```python
from build123d import *

# Parameters (mm, degrees)
CROQUIS1_W              = 237
CROQUIS1_H              = 450
SALIENTE_EXTRUIR1_DEPTH = 10
CROQUIS2_W              = 5
CROQUIS2_H              = 450
SALIENTE_EXTRUIR2_DEPTH = 70
CROQUIS3_R              = 2
CORTAR_EXTRUIR1_DEPTH   = 70
CROQUIS4_W              = 450
CROQUIS4_H              = 70
CORTAR_EXTRUIR2_DEPTH   = 10
CROQUIS5_R              = 10
CORTAR_EXTRUIR4_DEPTH   = 10


with BuildPart() as part:
    # Croquis1 → Saliente-Extruir1 (new body)
    with BuildSketch(Plane(origin=(0, 0, 0), x_dir=(1, 0, 0), z_dir=(0, 1, 0))):
        Rectangle(CROQUIS1_W, CROQUIS1_H)
    extrude(amount=SALIENTE_EXTRUIR1_DEPTH)

    # Croquis2 → Saliente-Extruir2 (add)
    with BuildSketch(Plane.XZ):
        with Locations((-116, 0)):
            Rectangle(CROQUIS2_W, CROQUIS2_H)
    extrude(amount=SALIENTE_EXTRUIR2_DEPTH)

    # Croquis3 → Cortar-Extruir1 (cut)
    with BuildSketch(Plane(origin=(-113.5, 0, 0), x_dir=(0, 0, -1), z_dir=(1, 0, 0))):
        with Locations((-215, -10)):
            Circle(CROQUIS3_R)
        with Locations((215, -10)):
            Circle(CROQUIS3_R)
        with Locations((215, -60)):
            Circle(CROQUIS3_R)
        with Locations((-215, -60)):
            Circle(CROQUIS3_R)
    extrude(amount=-CORTAR_EXTRUIR1_DEPTH, mode=Mode.SUBTRACT)

    # Croquis4 → Cortar-Extruir2 (cut)
    with BuildSketch(Plane(origin=(-113.5, 0, 0), x_dir=(0, 0, -1), z_dir=(1, 0, 0))):
        with Locations((0, -35)):
            Rectangle(CROQUIS4_W, CROQUIS4_H)
    extrude(amount=-CORTAR_EXTRUIR2_DEPTH, mode=Mode.SUBTRACT)

    # Croquis5 → Cortar-Extruir4 (cut)
    with BuildSketch(Plane.XZ):
        with Locations((-98.5, 35.8)):
            Circle(CROQUIS5_R)
    extrude(amount=-CORTAR_EXTRUIR4_DEPTH, mode=Mode.SUBTRACT)


solid = part.part
```
Build history of the part. All positions in model axes, mm. Coordinates: 2 decimals unless noted, no trailing zeros. Write each loop counter-clockwise with the first axis right and the second up, starting at its lowest first coordinate (ties: lowest second). Pieces come first, ordered by that corner, then holes.
1. Band-saw the part on B-B, the plane x = -98.5. Give the cut face in (y, z), and give its area (3 significant figures).
Answer block:
outline: (0, -225) - (10, -225) - (10, 25.8) - (0, 25.8) - close; (0, 45.8) - (10, 45.8) - (10, 225) - (0, 225) - close
area: 4,300 mm2
2. Pull direction Z, two halves, no side cores. Call faces 1 (the flat face through (-2, 5, -225)), 2 (the cylindrical face through (-105.87, 4.93, 42.56)), 3 (the flat face through (-2, 10, -3)): released by +Z, released by -Z, zero draft, split by the parting line, or undercut.
Answer block:
face 1: released by -Z
face 2: undercut
face 3: zero draft
3. Drill centre line: probe 1 along Z at (x, y) = (-98.5, 5.75). Where is it in solid material? Low to high.
Answer block:
probe 1: z = -225 to 25.8, 45.8 to 225
4. Band-saw the part on A-A, the plane z = 35.8. Give the cut face in (x, y), and give its area (3 significant figures).
Answer block:
outline: (-118.5, 0) - (-108.5, 0) - (-108.5, 10) - (-118.5, 10) - close; (-88.5, 0) - (118.5, 0) - (118.5, 10) - (-88.5, 10) - close
area: 2,170 mm2
5. Drop flat-ended pins along their axis: pin 1 (4 mm diameter, centred on x = -14.5, z = 20, fed in from -Y); pin 2 (18 mm diameter, centred on x = -98.5, z = 35.8, fed in from -Y). Give the stop position or say it passes through.
Answer block:
pin 1: stops at y = 0
pin 2: passes through
